```python
from build123d import *


with BuildPart() as f1:
    # F0 (on Right) → F1 (revolve)
    with BuildSketch(Plane.YZ):
        Polygon((-20, 125), (-37.5, 125), (-37.5, 82.5), (-17.558118, 82.5), (-17.558118, 37.5), (-50, 37.5), (-50, 12.5), (0, 12.5), (50, 12.5), (50, 37.5), (17.558118, 37.5), (17.558118, 82.5), (37.5, 82.5), (37.5, 125), (20, 125), (20, 100), (0, 100), (-20, 100), align=None)
    revolve(axis=Axis((0, -4.137259, 0), (0, 1, 0)))


solid = f1.part
```
Can you work these out from the model? Positions are in its coordinate system, mm. A direction names the side the tool comes from. Round coordinates to 2 decimals unless told otherwise and drop trailing zeros. Order: outer loops, then holes, each group sorted by start corner. A loop starts at its lowest first (then second) coordinate and runs counter-clockwise, first axis right, second up. Notation, with made-up numbers: (9, 84.5) -> (14, 84.5) arc R21 cw to (14, 114.5) -> close; hole circle Ø7 at (41.5, 62). An arc over 180 degrees is marked (long way). Return JSON: item names as keys, results as strings. Group by question number.
1. We'd pull the mould along Y, two halves only. Please class faces 1 (the face through (-26, 37.5, -82)), 2 (the face through (3.755, 0.7, 11.923)), 3 (the face through (30.04, -0.28, 95.38)): released by +Y, released by -Y, zero draft, split by the parting line, or undercut.
2. I need wall thicknesses on line 1 (X direction, y = 24.5, z = 0); line 2 (X direction, y = 1, z = 0); line 3 (Y direction, x = 114, z = -3.5). Which ranges of each line are inside material? Lowest first, please. Write a range as [from, to].
3. Will these pins go through, and if not, where does the flat tip stop? pin 1 (6 mm diameter, centred on x = 25.5, y = -23.5, fed in from +Z); pin 2 (6 mm diameter, centred on x = 93.5, z = 6.5, fed in from +Y); pin 3 (5 mm diameter, centred on x = -23, z = -71, fed in from -Y).
4. If we section it at D-D, the plane x = 46: Write out the boundary of the cut face in (y, z), then the cut area to 3 significant figures.
5. If we section it at C-C, the plane y = -26.5: Write out the boundary of the cut face in (x, z), then the cut area to 3 significant figures.
6. Which directions (+Z, -Z, +X, -X, +Y, -Y) give clear straight access to the entire face, cutting with the end or side of a thin tool? Please do faces 4 (the face through (-80.54, 27.67, -17.88)), 5 (the face through (37.18, -34.01, -4.88)), 6 (the face through (5.5, -28.87, -124.88)), 7 (the face through (84, 20, -56)).
Output values:
{
 "1": {"face 1": "released by +Y", "face 2": "zero draft", "face 3": "undercut"},
 "2": {"line 1": "[-125, -82.5], [-37.5, -12.5], [12.5, 37.5], [82.5, 125]", "line 2": "[-100, -12.5], [12.5, 100]", "line 3": "[-37.5, -20], [20, 37.5]"},
 "3": {"pin 1": "z = 122.96", "pin 2": "y = 37.5", "pin 3": "y = -17.56"},
 "4": {"outline": "(-37.5, -116.23) -> (-20, -116.23) -> (-20, -88.79) -> (20, -88.79) -> (20, -116.23) -> (37.5, -116.23) -> (37.5, -68.49) -> (17.56, -68.49) -> (17.56, 68.49) -> (37.5, 68.49) -> (37.5, 116.23) -> (20, 116.23) -> (20, 88.79) -> (-20, 88.79) -> (-20, 116.23) -> (-37.5, 116.23) -> (-37.5, 68.49) -> (-17.56, 68.49) -> (-17.56, -68.49) -> (-37.5, -68.49) -> close", "area": "9,780 mm²"},
 "5": {"outline": "circle Ø250 at (0, 0); circle Ø75 at (0, 0); hole circle Ø165 at (0, 0); hole circle Ø25 at (0, 0)", "area": "31,600 mm²"},
 "6": {"face 4": "+Y", "face 5": "-Y", "face 6": "+Y, -Y", "face 7": "none"}
}
